Check sheet for the drawn part. Datum: minimum x, y, z corner. Units: mm. Coordinates: 2 decimals unless noted, no trailing zeros. Loops run counter-clockwise (first coordinate to the right, second up) from the corner with the lowest first, then second, coordinate; pieces in that order, holes last.
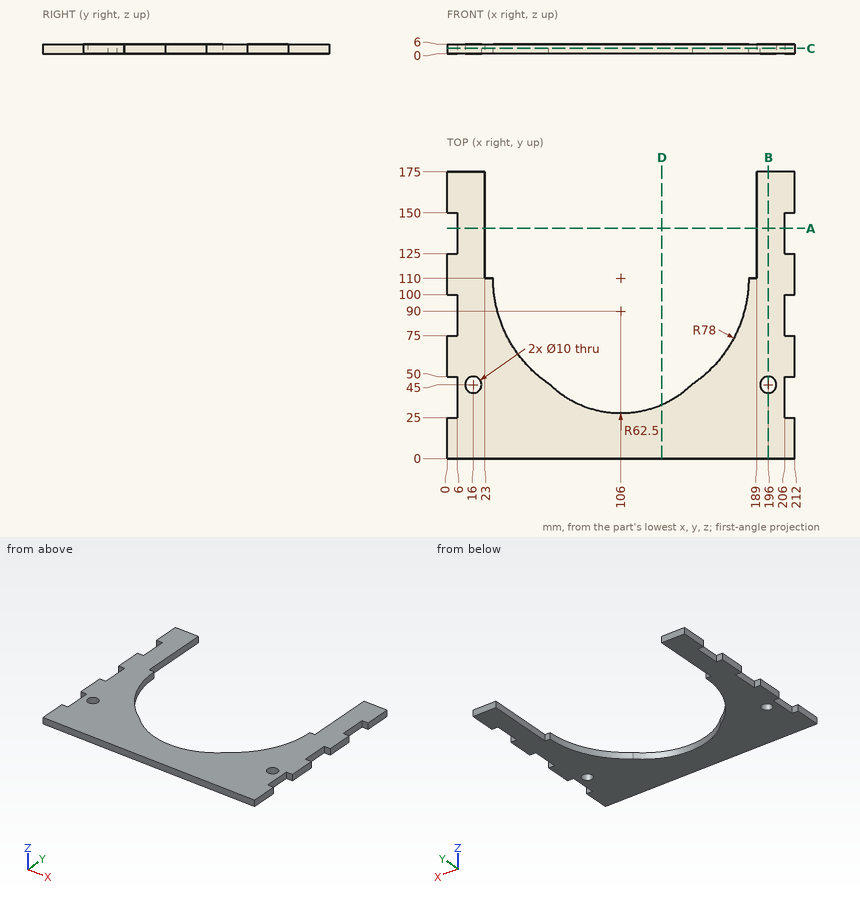
1) Section check D-D on x = 131. Enter the section's corners in (y, z).
Answer sheet:
outline: (0, 0) - (32.72, 0) - (32.72, 6) - (0, 6) - close
2) Section check A-A on y = 140.5. Enter the section's corners in (x, z), plus the area to 3 significant figures.
Answer sheet:
outline: (6, 0) - (23, 0) - (23, 6) - (6, 6) - close; (189, 0) - (206, 0) - (206, 6) - (189, 6) - close
area: 204 mm2
3) Section check C-C on z = 3.3. Give the number of separate pieces and of enclosed holes in the cut face, plus the area to 3 significant figures.
Answer sheet:
separate pieces: 1
enclosed holes: 2
area: 15,400 mm2
4) Scan lines: line 1 (Y direction, x = 16, z = 2.6); line 2 (X direction, y = 162.5, z = 1.5); line 3 (X direction, y = 82, z = 4.4). Record each from-to range of solid material in increasing order.
Answer sheet:
line 1: y = 0 to 40, 50 to 175
line 2: x = 0 to 23, 189 to 212
line 3: x = 6 to 33.2, 178.8 to 206
5) Section check B-B on x = 196. Enter the section's corners in (y, z), plus the area to 3 significant figures.
Answer sheet:
outline: (0, 0) - (40, 0) - (40, 6) - (0, 6) - close; (50, 0) - (175, 0) - (175, 6) - (50, 6) - close
area: 990 mm2
6) Depth check by flat-ended pin: pin 1 (3 mm diameter, centred on y = 34, z = 3, fed in from -X). Enter the tip coordinate at first touch or a pass-through.
Answer sheet:
pin 1: stops at x = 6
